Design review of the part built by this model. Coordinates are the model's own, in mm. A direction names the side the tool comes from. Coordinates: 2 decimals unless noted, no trailing zeros. Loops run counter-clockwise (first coordinate to the right, second up) from the corner with the lowest first, then second, coordinate; pieces in that order, holes last. Notation, with made-up numbers: M 39,20 L 44,20 A11 ccw 44,26 Z; hole C 87.5,37 d8. An arc over 180 degrees is marked long. One line per item, written item: value.
Autodesk Fusion 360 part; units mm, degrees
sketch "Sketch1" plane through (0, 0, 0) normal (0, 0, 1) x (1, 0, 0)
  circle A0 centre (0, 0) radius 9.75
  line L0 (0.0224, 9.75) -> (0.0224, 24.75)
  line L1 (0.0224, 24.75) -> (-19.9776, 24.75)
  line L2 (-19.9776, 24.75) -> (-19.9776, -24.75)
  line L3 (-19.9776, -24.75) -> (0, -24.75)
  line L4 (0, -24.75) -> (0, -9.75)
  line L5 (0, -24.75) -> (6.5, -24.75) construction
  line L6 (0, -24.75) -> (-6.5, -24.75) construction
  line L7 (-6.5, -24.75) -> (-6.5, -46.75)
  line L8 (-6.5, -46.75) -> (12.5, -46.75)
  line L9 (12.5, -46.75) -> (12.5, -25)
  line L10 (-6.5, -24.75) -> (-12.5, -24.75)
  line L11 (-12.5, -24.75) -> (-12.5, -46.75)
  line L12 (0, -24.75) -> (12.5, -24.75)
  line L13 (12.5, -24.75) -> (12.5, -25)
  line L14 (-6.5, -46.75) -> (-12.5, -46.75)
  dimension "d1" = 19.5
  dimension "d2" = 15
  dimension "d3" = 20
  dimension "d4" = 49.5
  dimension "d5" = 6.5
  dimension "d6" = 6.5
  dimension "d7" = 22
  dimension "d8" = 19
  dimension "d9" = 6
extrude "Extrude1" add sketch "Sketch1" along normal blind 40 contours A0 L0 L1 L2 L3 L4 L10
extrude "Extrude2" add sketch "Sketch1" along normal blind 13.6 contours L3 L7 L8 L9 L12 L13
extrude "Extrude3" add sketch "Sketch1" along normal blind 26.4 contours L3 L7 L10 L11 L14
sketch "Sketch2" plane through (-19.9776, 0, 0) normal (-1, 0, 0) x (0, -1, 0)
  line L0 (-24.75, 0) -> (24.75, 0)
  line L1 (24.75, 0) -> (24.75, 40)
  line L2 (24.75, 40) -> (-24.75, 40)
  line L3 (-24.75, 40) -> (-24.75, 0)
  line L4 (0, 40) -> (-9.75, 40) construction
  line L5 (-24.75, 40) -> (-17.25, 40) construction
  line L6 (-17.25, 40) -> (-17.25, 30) construction
  circle A0 centre (-17.25, 30) radius 2.5
  circle A1 centre (17.25, 30) radius 2.5
  circle A2 centre (-17.25, 10) radius 2.5
  circle A3 centre (17.25, 10) radius 2.5
  dimension "d16" = 9.75
  dimension "d17" = 7.5
  dimension "d18" = 10
  dimension "d20" = 5
  dimension "d23" = 34.5
  dimension "d24" = -20
extrude "Extrude4" cut sketch "Sketch2" against normal blind 30 contours A0 | A1 | A2 | A3
sketch "Sketch3" plane through (0, 0, 13.6) normal (0, 0, 1) x (-1, 0, 0)
  line L0 (6.5, 24.75) -> (6.5, 46.75)
  line L1 (6.5, 46.75) -> (-12.5, 46.75)
  line L2 (-12.5, 46.75) -> (-12.5, 25)
  line L3 (0, 24.75) -> (6.5, 24.75)
  line L4 (-12.5, 25) -> (-12.5, 24.75)
  line L5 (-12.5, 24.75) -> (0, 24.75)
  line L6 (0, 24.75) -> (0, 30.75) construction
  circle A0 centre (0, 30.75) radius 2.25
  circle A1 centre (0, 40.75) radius 2.25
  dimension "d28" = 6
  dimension "d29" = 4.5
  dimension "d32" = 0
  dimension "d33" = 10
extrude "Extrude5" cut sketch "Sketch3" against normal blind 14 contours A0 | A1
sketch "Sketch4" plane through (-19.9776, 0, 0) normal (-1, 0, 0) x (0, -1, 0)
  circle A0 centre (17.25, 30) radius 2.5
  circle A1 centre (17.25, 10) radius 2.5
  circle A2 centre (-17.25, 30) radius 2.5
  circle A3 centre (-17.25, 10) radius 2.5
  line L0 (-24.75, 0) -> (24.75, 0)
  line L1 (24.75, 0) -> (24.75, 40)
  line L2 (24.75, 40) -> (-24.75, 40)
  line L3 (-24.75, 40) -> (-24.75, 0)
  line L4 (0, 40) -> (0, 0) construction
  circle A4 centre (0, 20) radius 2.5
  dimension "d36" = 5
extrude "Extrude6" cut sketch "Sketch4" against normal blind 20 contours A4
sketch "Sketch5" plane through (-19.9776, 0, 0) normal (-1, 0, 0) x (0, -1, 0)
  circle A0 centre (0, 20) radius 2.5
  circle A1 centre (17.25, 30) radius 2.5
  circle A2 centre (17.25, 10) radius 2.5
  circle A3 centre (-17.25, 30) radius 2.5
  circle A4 centre (-17.25, 10) radius 2.5
  line L0 (-24.75, 0) -> (24.75, 0)
  line L1 (24.75, 0) -> (24.75, 40)
  line L2 (24.75, 40) -> (-24.75, 40)
  line L3 (-24.75, 40) -> (-24.75, 0)
  line L4 (0, 20) -> (2.5, 24.3301) construction
  line L5 (0, 20) -> (5, 20) construction
  line L6 (0, 20) -> (-2.5, 24.3301) construction
  line L7 (0, 20) -> (5, 20) construction
  line L8 (0, 20) -> (-5, 20) construction
  line L9 (0, 20) -> (2.5, 15.6699) construction
  line L10 (-2.5, 15.6699) -> (0, 20) construction
  line L11 (5, 20) -> (2.5, 15.6699)
  line L12 (2.5, 15.6699) -> (-2.5, 15.6699)
  line L13 (-2.5, 15.6699) -> (-5, 20)
  line L14 (-5, 20) -> (-2.5, 24.3301)
  line L15 (-2.5, 24.3301) -> (2.5, 24.3301)
  line L16 (2.5, 24.3301) -> (5, 20)
  dimension "d40" = 60
  dimension "d41" = 5
  dimension "d42" = 120
  dimension "d43" = 5
  dimension "d44" = 5
  dimension "d45" = 5
extrude "Extrude7" cut sketch "Sketch5" against normal blind 7 from surface at -6 contours L11 L12 L13 L14 L15 L16
sketch "Sketch6" plane through (-19.9776, 0, 0) normal (-1, 0, 0) x (0, -1, 0)
  circle A0 centre (0, 20) radius 2.5
  circle A1 centre (17.25, 30) radius 2.5
  circle A2 centre (17.25, 10) radius 2.5
  circle A3 centre (-17.25, 30) radius 2.5
  circle A4 centre (-17.25, 10) radius 2.5
  line L0 (-24.75, 0) -> (24.75, 0)
  line L1 (24.75, 0) -> (24.75, 40)
  line L2 (24.75, 40) -> (-24.75, 40)
  line L3 (-24.75, 40) -> (-24.75, 0)
  circle A5 centre (-17.25, 30) radius 5
  circle A6 centre (17.25, 30) radius 5
  circle A7 centre (-17.25, 10) radius 5
  circle A8 centre (17.25, 10) radius 5
  dimension "d49" = 10
  dimension "d52" = 34.5
  dimension "d53" = -20
extrude "Extrude8" cut sketch "Sketch6" against normal blind 3 contours A5 | A6 | A7 | A8
fillet "Fillet1" radius 2.5 1 edges at (-12.5, -24.75, 13.2)
(1) We need section C-C on x = -3.5. State the section outline as (y, z) points, then the cut area to 3 significant figures.
Reply:
outline: M -46.75,0 L -9.1,0 L -9.1,40 L -24.75,40 L -24.75,13.6 L -46.75,13.6 Z; M 9.1,0 L 24.75,0 L 24.75,40 L 9.1,40 Z; hole C -17.25,10 d5; hole C -17.25,30 d5; hole C 17.25,10 d5; hole C 17.25,30 d5
area: 1,470 mm2
(2) We need section B-B on y = 17.25. State the section outline as (x, z) points, then the cut area to 3 significant figures.
Reply:
outline: M -19.98,0 L 0.02,0 L 0.02,7.5 L -16.98,7.5 L -16.98,5 L -19.98,5 Z; M -19.98,15 L -16.98,15 L -16.98,12.5 L 0.02,12.5 L 0.02,27.5 L -16.98,27.5 L -16.98,25 L -19.98,25 Z; M -19.98,35 L -16.98,35 L -16.98,32.5 L 0.02,32.5 L 0.02,40 L -19.98,40 Z
area: 570 mm2
(3) We need section A-A on y = 0. State the section outline as (x, z) points, then the cut area to 3 significant figures.
Reply:
outline: M -19.98,0 L -9.75,0 L -9.75,15.67 L -13.98,15.67 L -13.98,17.5 L -19.98,17.5 Z; M -19.98,22.5 L -13.98,22.5 L -13.98,24.33 L -9.75,24.33 L -9.75,40 L -19.98,40 Z
area: 342 mm2
(4) Tool access review of faces 5 (the cylindrical face through (-18.5, 18.33, 25.12)), 6 (the cylindrical face through (-17.02, 0.33, 22.48)), 7 (the flat face through (-11.21, -3.73, 22.2)), 8 (the flat face through (3, -36, 13.6)), 9 (the flat face through (-12.5, -37, 13)): name each direction out of +Z, -Z, +X, -X, +Y, -Y from which nothing blocks a thin tool from reaching the whole face with its end or side.
Reply:
face 5: -X
face 6: +X, -X
face 7: +X
face 8: +Z, +X, -Y
face 9: +Z, -Z, -X, -Y
(5) We need section D-D on z = 4. State the section outline as (x, y) points, then the cut area to 3 significant figures.
Reply:
outline: M -19.98,-24.75 L -15,-24.75 A2.5 cw -12.5,-27.25 L -12.5,-46.75 L 12.5,-46.75 L 12.5,-24.75 L 0,-24.75 L 0,-9.75 A9.75 cw 0.02,9.75 L 0.02,24.75 L -19.98,24.75 Z; hole C 0,-40.75 d4.5; hole C 0,-30.75 d4.5
area: 1,360 mm2
(6) Mouldability with a two-part tool opening along Z and no side actions: class faces 1 (the cylindrical face through (-18.5, -16.17, 25.12)), 2 (the flat face through (0, -17, 20)), 3 (the flat face through (-8, -10, 0)), 4 (the flat face through (-16.978, 20, 9)) as released by +Z, released by -Z, zero draft, split by the parting line, or undercut.
Reply:
face 1: undercut
face 2: zero draft
face 3: released by -Z
face 4: undercut
(7) Insertion check: pin 1 (8 mm diameter, centred on y = 17.25, z = 10, fed in from +X); pin 2 (4.5 mm diameter, centred on y = -17.25, z = 10, fed in from -X); pin 3 (7 mm diameter, centred on x = 0, y = -40.75, fed in from +Z); pin 4 (6.5 mm diameter, centred on y = -33, z = 18.5, fed in from +X). Each pin has a flat end and moves straight along its axis. Give the tip position at first contact, or say it passes through.
Reply:
pin 1: stops at x = 0.02
pin 2: passes through
pin 3: stops at z = 13.6
pin 4: stops at x = -6.5
(8) To check wall thickness, follow line 1 along Z through (x, y) = (-18, 17); line 2 along X through (y, z) = (-41, 10); line 3 along Y through (x, z) = (-12, 32). State the ranges of each line that lie inside material, in increasing order. Write a range as [from, to].
Reply:
line 1: z = [0, 5.01], [14.99, 25.01], [34.99, 40]
line 2: x = [-12.5, -2.24], [2.24, 12.5]
line 3: y = [-24.75, -18.75], [-15.75, 15.75], [18.75, 24.75]
